from build123d import *

# Parameters (mm, degrees)
ESBO_O1_W                = 2
ESBO_O1_H                = 8
ESBO_O1_R                = 3
ESBO_O1_R_2              = 2.5
RESSALTO_EXTRUS_O1_DEPTH = 10
ESBO_O4_W                = 4
ESBO_O4_H                = 3.861250687
ESBO_O4_H_2              = 3.752003841
ESBO_O4_W_2              = 5
ESBO_O4_H_3              = 3.819014792
ESBO_O4_H_4              = 3.693699436
ESBO_O4_W_3              = 1.5
ESBO_O4_H_5              = 2.079089953
CORTE_EXTRUS_O1_DEPTH    = 10
ESBO_O5_R                = 1.5
CORTE_EXTRUS_O2_DEPTH    = 10


with BuildPart() as part:
    # Esboço1 → Ressalto-extrusão1 (new body)
    with BuildSketch(Plane.XY):
        with BuildLine():
            Line((-25.719653684, -5.942716093), (-16.131983613, -5.942716093))
            Line((-16.131983613, -5.942716093), (7.368016387, -5.942716093))
            Line((7.368016387, -5.942716093), (16.955686457, -5.942716093))
            ThreePointArc((16.955686457, -5.942716093), (18.455686457, -4.442716093), (16.955686457, -2.942716093))
            add(Edge.make_bspline(
                [(12.952874444, 0), (12.912537119, -1.482141434), (14.266501813, -2.619700333), (15.801098565, -2.968716739), (16.955686457, -2.942716093)],
                knots=[0, 0, 0, 0, 0.504814455, 1, 1, 1, 1], degree=3))
            add(Edge.make_bspline(
                [(12.952874444, 0), (12.309204111, 4.600095009), (7.368016387, 4.358240851)],
                knots=[0, 0, 0, 1, 1, 1], degree=2))
            Line((7.368016387, 4.358240851), (-12.64298655, 4))
            add(Edge.make_bspline(
                [(-12.64298655, 4), (-13.901476132, 4.065275886), (-14.043723736, 5.271225486), (-15.883550882, 5.59671809), (-16.925443363, 5.584858058)],
                knots=[0, 0, 0, 0, 0.56422845, 1, 1, 1, 1], degree=3))
            ThreePointArc((-16.925443363, 5.584858058), (-20.354846171, 3.679270895), (-21.716841671, 0))
            add(Edge.make_bspline(
                [(-21.716841671, 0), (-21.676504345, -1.482141434), (-23.030469039, -2.619700333), (-24.565065791, -2.968716739), (-25.719653684, -2.942716093)],
                knots=[0, 0, 0, 0, 0.504814455, 1, 1, 1, 1], degree=3))
            ThreePointArc((-25.719653684, -2.942716093), (-27.219653684, -4.442716093), (-25.719653684, -5.942716093))
        make_face()
        with Locations((-17.066284799, 0)):
            Rectangle(ESBO_O1_W, ESBO_O1_H, mode=Mode.SUBTRACT)
        with Locations((-12.066284799, 0)):
            Circle(ESBO_O1_R, mode=Mode.SUBTRACT)
        with Locations((-5.066284799, 0)):
            Circle(ESBO_O1_R, mode=Mode.SUBTRACT)
        with Locations((1.433715201, 0)):
            Circle(ESBO_O1_R_2, mode=Mode.SUBTRACT)
        with Locations((7.433715201, 0)):
            Circle(ESBO_O1_R_2, mode=Mode.SUBTRACT)
    extrude(amount=RESSALTO_EXTRUS_O1_DEPTH)

    # Esboço4 → Corte-extrusão1 (cut)
    with BuildSketch(Plane(origin=(0, 0, 0), x_dir=(-1, 0, 0), z_dir=(0, 0, -1))):
        with Locations((-7.433715201, 3.430625344)):
            Rectangle(ESBO_O4_W, ESBO_O4_H)
        with Locations((-1.433715201, 3.376001921)):
            Rectangle(ESBO_O4_W, ESBO_O4_H_2)
        with Locations((5.066284799, 3.567819791)):
            Rectangle(ESBO_O4_W_2, ESBO_O4_H_3)
        with Locations((12.066284799, 3.505162113)):
            Rectangle(ESBO_O4_W_2, ESBO_O4_H_4)
        with Locations((17.066284799, 4.780683053)):
            Rectangle(ESBO_O4_W_3, ESBO_O4_H_5)
    extrude(amount=-CORTE_EXTRUS_O1_DEPTH, mode=Mode.SUBTRACT)

    # Esboço5 → Corte-extrusão2 (cut)
    with BuildSketch(Plane(origin=(0, 0, 0), x_dir=(1, 0, 0), z_dir=(0, 1, 0))):
        with Locations(Location((-24.219653684, -5, 0), (0, 0, 180))):
            Circle(ESBO_O5_R)
        with Locations((15.455686457, -5)):
            Circle(ESBO_O5_R)
    extrude(amount=-CORTE_EXTRUS_O2_DEPTH, mode=Mode.SUBTRACT)


solid = part.part
Can you work these out from the model? Positions are in its coordinate system, mm. A direction names the side the tool comes from. Give positions to 0.01 mm unless a question says otherwise; leave off trailing zeros. One line per item, written item: value. Start each with the question number.
1) If I drill on line 1 (X direction, y = -4.25, z = 6.25); line 2 (X direction, y = -5.15, z = 5); line 3 (X direction, y = 2.75, z = 5.5), over which ranges is the centre line in solid material (lowest first)? Write a range as [from, to].
2) On a 3-axis mill with a long thin cutter (end or side, diameter ignored), from which of +Z, -Z, +X, -X, +Y, -Y can I reach the whole of each face in a straight line? I mean faces 4 (the face through (-17, -4, 5)), 5 (the face through (-16.316, 5, 5)), 6 (the face through (-22.72, -4.47, 5.07)). Say none if no direction works.
3) Thinking about a two-plate mould opening in Y: for faces 1 (the face through (13.957, -4.467, 4.934)), 2 (the face through (-12, -3, 5)), 3 (the face through (18.455, -4.476, 4.93)), which applies, +Y half, -Y half, draft (parallel to the pull), parting line (faces both ways), or undercut?
4) I'm going to push flat-ended pins straight in: pin 1 (1.5 mm diameter, centred on y = 4.5, z = 4.5, fed in from +X); pin 2 (1.5 mm diameter, centred on y = 0, z = 5.5, fed in from +X); pin 3 (2 mm diameter, centred on y = 3, z = 3, fed in from +X). Where does each tip first touch, or does it pass through?
Completed:
1. line 1: x = [-27.21, -25.05], [-23.39, 14.63], [16.28, 18.44]
1. line 2: x = [-27.04, -25.72], [-22.72, 13.96], [16.96, 18.28]
1. line 3: x = [-21, -18.07], [-16.07, -14.57], [-9.57, -7.57], [-2.57, -0.57], [3.43, 5.43], [9.43, 11.88]
2. face 4: +Z, -Z
2. face 5: +Z, -Z, +Y
2. face 6: +Y, -Y
3. face 1: draft
3. face 2: undercut
3. face 3: parting line
4. pin 1: stops at x = 10.68
4. pin 2: stops at x = 13
4. pin 3: stops at x = 12.36
